The listing builds one solid part. Answer for the finished solid, in the listing's coordinates (mm). A direction names the side the tool comes from. Coordinates: 2 decimals unless noted, no trailing zeros. Write each loop counter-clockwise with the first axis right and the second up, starting at its lowest first coordinate (ties: lowest second). Pieces come first, ordered by that corner, then holes.
(1) Which of the six approach directions +Z, -Z, +X, -X, +Y, -Y give full straight-line access (tool end or side, diameter ignored) to faces 1 (the flat face through (69, 0, 86.754)), 2 (the cylindrical face through (46.441, 2.068, 74.532)), 3 (the flat face through (65.98, 0, 54)), 4 (the flat face through (23, 0, 76.163)), 5 (the flat face through (30.556, 0, 100))?
(2) The part is cut by section C-C on z = 83.5. Determine the outline of the cut face in (x, y), plus the area to 3 significant figures.
(3) Straight lines are drawn through the part: line 1 (Z direction, x = 24.5, y = -3.5); line 2 (Z direction, x = 69, y = 0.5); line 3 (X direction, y = 3, z = 54.5). For each, find the intervals that lie inside material, in ascending order.
(4) The part is cut by section A-A on x = 57.5. Determine the outline of the cut face in (y, z), plus the area to 3 significant figures.
(5) The part is cut by section B-B on z = 78. Determine the outline of the cut face in (x, y).
(6) Given P1, Ø3.5, axis at x = 33.5, y = 1, coming from the -Z side; P2, Ø1.4, axis at y = -1, z = 64.5, coming from the -X side; P3, Ø3.5, axis at x = 47, z = 77.5, coming from the +Y side, each flat-ended and moving along its own axis, determine where each tip first touches the part or whether it passes through.
(7) For a pull along X with two mould halves and no side action, classify faces 6 (the flat face through (25.34, 0, 54)), 7 (the flat face through (33, 0, 55.843)), 8 (the flat face through (38, 0, 51.194)) as +X half, -X half, draft (parallel to the pull), parting line (faces both ways), or undercut.
from build123d import *

# Parameters (mm, degrees)
SKETCH3_W                = 50.8
SKETCH3_H                = 50.8
BOSS_EXTRUDE5_DEPTH      = 4.572
BOSS_EXTRUDE5_DEPTH_BACK = 4.5212
SKETCH4_W                = 4.6482
SKETCH4_H                = 4.6482
CUT_EXTRUDE4_DEPTH       = 9.0932
SKETCH10_R               = 3.280660975
CUT_EXTRUDE9_DEPTH       = 5.08
SKETCH9_W                = 4.6482
SKETCH9_H                = 4.6482
CUT_EXTRUDE10_DEPTH      = 9.144
LPATTERN1_COUNT          = 5
LPATTERN1_PITCH          = 10.16
LPATTERN2_COUNT          = 5
LPATTERN2_PITCH          = 10.16
LPATTERN3_COUNT          = 5
LPATTERN3_PITCH          = 10.16
SKETCH13_W               = 4.6482
SKETCH13_H               = 4.6482
CUT_EXTRUDE11_DEPTH      = 9.144
LPATTERN4_COUNT          = 4
LPATTERN4_PITCH          = 10.16


with BuildPart() as part:
    # Sketch3 → Boss-Extrude5 (new body, two sides)
    with BuildSketch(Plane(origin=(0, 0, 0), x_dir=(1, 0, 0), z_dir=(0, 1, 0))) as boss_extrude5_sk:
        with Locations((46.091507602, -76.594393473)):
            Rectangle(SKETCH3_W, SKETCH3_H)
    extrude(amount=BOSS_EXTRUDE5_DEPTH)
    extrude(boss_extrude5_sk.sketch, amount=-BOSS_EXTRUDE5_DEPTH_BACK)

    # Sketch4 → Cut-Extrude4 (cut)
    with BuildSketch(Plane(origin=(0, 4.572, 0), x_dir=(1, 0, 0), z_dir=(0, 1, 0))):
        with Locations((23.015607602, -53.518493473)):
            Rectangle(SKETCH4_W, SKETCH4_H)
    cut_extrude4 = extrude(amount=-CUT_EXTRUDE4_DEPTH, mode=Mode.SUBTRACT)

    # Sketch10 → Cut-Extrude9 (cut)
    with BuildSketch(Plane(origin=(0, 4.572, 0), x_dir=(1, 0, 0), z_dir=(0, 1, 0))):
        with Locations(Location((46.297206245, -77.809978732, 0), (0, 0, 270))):  # turned: the seam where the file's is
            Circle(SKETCH10_R)
    extrude(amount=-CUT_EXTRUDE9_DEPTH, mode=Mode.SUBTRACT)

    # Sketch9 → Cut-Extrude10 (cut)
    with BuildSketch(Plane(origin=(0, 4.572, 0), x_dir=(1, 0, 0), z_dir=(0, 1, 0))):
        with Locations((69.167407602, -58.59849342)):
            Rectangle(SKETCH9_W, SKETCH9_H)
    cut_extrude10 = extrude(amount=-CUT_EXTRUDE10_DEPTH, mode=Mode.SUBTRACT)

    # LPattern1: Cut-Extrude4 ×5
    with Locations(*[(0, 0, i * LPATTERN1_PITCH) for i in range(1, LPATTERN1_COUNT)]):
        add(cut_extrude4, mode=Mode.SUBTRACT)

    # LPattern2: Cut-Extrude10 ×5
    with Locations(*[(0, 0, i * LPATTERN2_PITCH) for i in range(1, LPATTERN2_COUNT)]):
        add(cut_extrude10, mode=Mode.SUBTRACT)

    # LPattern3: Cut-Extrude4 ×5
    with Locations(*[(i * LPATTERN3_PITCH, 0, 0) for i in range(1, LPATTERN3_COUNT)]):
        add(cut_extrude4, mode=Mode.SUBTRACT)

    # Sketch13 → Cut-Extrude11 (cut)
    with BuildSketch(Plane(origin=(0, 4.572, 0), x_dir=(1, 0, 0), z_dir=(0, 1, 0))):
        with Locations((28.2321, -99.670293473)):
            Rectangle(SKETCH13_W, SKETCH13_H)
    cut_extrude11 = extrude(amount=-CUT_EXTRUDE11_DEPTH, mode=Mode.SUBTRACT)

    # LPattern4: Cut-Extrude11 ×4
    with Locations(*[(i * LPATTERN4_PITCH, 0, 0) for i in range(1, LPATTERN4_COUNT)]):
        add(cut_extrude11, mode=Mode.SUBTRACT)


solid = part.part
Model answer:
1. face 1: +X, +Y, -Y
1. face 2: +Y
1. face 3: -Z, +Y, -Y
1. face 4: -X, +Y, -Y
1. face 5: +Z, +Y, -Y
2. outline: (25.34, -4.52) - (71.49, -4.52) - (71.49, 4.57) - (25.34, 4.57) - close
2. area: 420 mm2
3. line 1: z = 55.84 to 61.35, 66 to 71.51, 76.16 to 81.67, 86.32 to 91.83, 96.48 to 101.99
3. line 2: z = 51.19 to 56.27, 60.92 to 66.43, 71.08 to 76.59, 81.24 to 86.75, 91.4 to 96.91, 101.56 to 101.99
3. line 3: x = 25.34 to 30.85, 35.5 to 41.01, 45.66 to 51.17, 55.82 to 61.33, 65.98 to 71.49
4. outline: (-4.52, 51.19) - (4.57, 51.19) - (4.57, 97.35) - (-4.52, 97.35) - close
4. area: 420 mm2
5. outline: (20.69, -4.52) - (66.84, -4.52) - (66.84, 4.57) - (49.57, 4.57) - (49.57, -0.51) - (43.02, -0.51) - (43.02, 4.57) - (20.69, 4.57) - close
6. P1: stops at z = 55.84
6. P2: stops at x = 25.34
6. P3: stops at y = -0.51
7. face 6: -X half
7. face 7: undercut
7. face 8: draft
